Work out the finished part from the listing and answer in its coordinate system (mm). A direction names the side the tool comes from. Give positions to 0.01 mm unless a question says otherwise; leave off trailing zeros. Loops run counter-clockwise (first coordinate to the right, second up) from the corner with the lowest first, then second, coordinate; pieces in that order, holes last. Notation, with made-up numbers: M 46.5,48.25 L 95.5,48.25 A32 ccw 95.5,75.25 Z; hole C 49.5,41 d4. An arc over 180 degrees is marked long. Answer in a Markdown table with one row per item. Add a question column.
from build123d import *

# Parameters (mm, degrees)
SALIENTE_EXTRUIR1_DEPTH = 9
CROQUIS2_R              = 1.875
CORTAR_EXTRUIR1_DEPTH   = 8.5
CROQUIS2_3_R            = 3.5
CROQUIS2_3_R_2          = 1.875
CORTAR_EXTRUIR2_DEPTH   = 2.8


with BuildPart() as part:
    # Croquis1 → Saliente-Extruir1 (new body)
    with BuildSketch(Plane(origin=(0, 0, 0), x_dir=(1, 0, 0), z_dir=(0, 1, 0))):
        with BuildLine():
            Line((16.75, 2), (25.53429067, 2))
            Line((25.53429067, 2), (43.53429067, 2))
            Line((43.53429067, 2), (43.53429067, 9.5))
            Line((43.53429067, 9.5), (32.645826686, 9.5))
            ThreePointArc((32.645826686, 9.5), (29.789462584, 16.388652139), (25.5, 22.488886144))
            Line((25.5, 22.488886144), (25.5, 31.304864393))
            Line((25.5, 31.304864393), (-25.5, 31.304864393))
            Line((-25.5, 31.304864393), (-25.5, 22.488886144))
            ThreePointArc((-25.5, 22.488886144), (-29.789462584, 16.388652139), (-32.645826686, 9.5))
            Line((-32.645826686, 9.5), (-43.53429067, 9.5))
            Line((-43.53429067, 9.5), (-43.53429067, 2))
            Line((-43.53429067, 2), (-25.53429067, 2))
            Line((-25.53429067, 2), (-16.75, 2))
            Line((-16.75, 2), (-16.75, 26.402432196))
            Line((-16.75, 26.402432196), (16.75, 26.402432196))
            Line((16.75, 26.402432196), (16.75, 2))
        make_face()
    extrude(amount=SALIENTE_EXTRUIR1_DEPTH)

    # Croquis2 → Cortar-Extruir1 (cut, through all)
    with BuildSketch(Plane(origin=(0, 0, -9.5), x_dir=(-1, 0, 0), z_dir=(0, 0, -1))):
        with Locations((37.645, 4.5)):
            Circle(CROQUIS2_R)
        with Locations((-37.645, 4.5)):
            Circle(CROQUIS2_R)
    extrude(amount=-CORTAR_EXTRUIR1_DEPTH, mode=Mode.SUBTRACT)

    # Croquis2_3 → Cortar-Extruir2 (cut)
    with BuildSketch(Plane(origin=(0, 0, -9.5), x_dir=(-1, 0, 0), z_dir=(0, 0, -1))):
        with Locations((-37.645, 4.5)):
            Circle(CROQUIS2_3_R)
        with Locations((-37.645, 4.5)):
            Circle(CROQUIS2_3_R_2, mode=Mode.SUBTRACT)
        with Locations((37.645, 4.5)):
            Circle(CROQUIS2_3_R)
        with Locations((37.645, 4.5)):
            Circle(CROQUIS2_3_R_2, mode=Mode.SUBTRACT)
    extrude(amount=-CORTAR_EXTRUIR2_DEPTH, mode=Mode.SUBTRACT)


solid = part.part
(1) Consider line 1 along X through (y, z) = (8.5, -4); line 2 along X through (y, z) = (2, -24.25); line 3 along Z through (x, y) = (-14, 0.5). Determine where each line is inside the solid, lowest interval first. Write a range as from..to.
(2) Section A-A, the plane y = 4.5 is taken. State how many separate pieces and enclosed holes the cut face has, and give its area (3 significant figures).
(3) Section C-C, the plane z = -28.75 is taken. Determine the outline of the cut face in (x, y).
(4) Section D-D, the plane x = 15.5 is taken. Determine the outline of the cut face in (y, z), and give its area (3 significant figures).
(5) Each of these flat-tipped pins is pushed along its axis until it touches: P1, Ø3, axis at x = 2, y = 3, coming from the +Z side; P2, Ø4.5, axis at x = -40.5, y = 6, coming from the -Z side; P3, Ø4.5, axis at y = 5, z = -27.5, coming from the +X side. Where does it stop, or does it pass through?
(6) The mould has two halves that part along X. Classify faces 1 (the face through (-16.75, 4, -14)), 2 (the face through (-30, 4, -16)), 3 (the face through (-1, 0, -27)): pulls with the +X half, pulls with the -X half, needs draft (parallel to the pull), parting line crosses it, or undercut.
(7) Section B-B, the plane z = -17.5 is taken. Determine the outline of the cut face in (x, y), and give its area (3 significant figures).
(8) Which of the six approach directions +Z, -Z, +X, -X, +Y, -Y give full straight-line access (tool end or side, diameter ignored) to faces 4 (the face through (25.5, 4, -27)), 5 (the face through (16.75, 4, -14)), 6 (the face through (-34.15, 4.65, -8.12))?
Numbers:
| question | item | result |
|---|---|---|
| 1 | line 1 | x = -43.53..-16.75, 16.75..43.53 |
| 1 | line 2 | x = -25.5..-16.75, 16.75..25.5 |
| 1 | line 3 | z = -31.3..-26.4 |
| 2 | separate pieces | 3 |
| 2 | enclosed holes | 0 |
| 2 | area | 982 mm² |
| 3 | outline | M -25.5,0 L 25.5,0 L 25.5,9 L -25.5,9 Z |
| 4 | outline | M 0,-31.3 L 9,-31.3 L 9,-26.4 L 0,-26.4 Z |
| 4 | area | 44.1 mm² |
| 5 | P1 | stops at z = -26.4 |
| 5 | P2 | stops at z = -9.5 |
| 5 | P3 | stops at x = 25.5 |
| 6 | face 1 | undercut |
| 6 | face 2 | pulls with the -X half |
| 6 | face 3 | needs draft |
| 7 | outline | M -29.15,0 L -16.75,0 L -16.75,9 L -29.15,9 Z; M 16.75,0 L 29.15,0 L 29.15,9 L 16.75,9 Z |
| 7 | area | 223 mm² |
| 8 | face 4 | -Z, +X, +Y, -Y |
| 8 | face 5 | +Z, +Y, -Y |
| 8 | face 6 | -Z |
